Build history of the part. All positions in model axes, mm. A direction names the side the tool comes from. Round coordinates to 2 decimals unless told otherwise and drop trailing zeros. Order: outer loops, then holes, each group sorted by start corner. A loop starts at its lowest first (then second) coordinate and runs counter-clockwise, first axis right, second up. Notation, with made-up numbers: (17.25, -20.75) -> (22.25, -20.75) arc R19 ccw to (22.25, -2.75) -> close; hole circle Ø7 at (18, -37). An arc over 180 degrees is marked (long way). Use a Markdown table: item, result. Add a question column.
Item 1: Slice it at D-D, the plane z = 0. State how many separate pieces and enclosed holes the cut face has, plus the area to 3 significant figures.
Item 2: Probe L1, parallel to Z at x = -31.5, y = 0; L2, parallel to Z at x = 34, y = -15; L3, parallel to Y at x = 30.5, z = 2. List the from-to ranges inside material, lowest first.
Item 3: Two-plate mould, pull along Z, no slides. Class faces 5 (the face through (0, -5, -21)), 6 (the face through (-41, 20, -6)), 7 (the face through (37, 3, -3)): released by +Z, released by -Z, zero draft, split by the parting line, or undercut.
Item 4: Slice it at B-B, the plane y = -15. Give the cut face in (x, z).
Item 5: Slice it at A-A, the plane x = 35. Give the cut face in (y, z).
Item 6: 3-axis set-ups, long thin cutter, end or side, ignore diameter. For faces 1 (the face through (1.02, -4.59, -18.97)), 2 (the face through (31, -13, -4)), 3 (the face through (25, 0, 0)), 4 (the face through (-25, 0, 0)): which of +Z, -Z, +X, -X, +Y, -Y reach the whole face in a straight line?
Item 7: Pin check, flat tips, straight feed: pin 1 (4 mm diameter, centred on x = 35, z = 0, fed in from +Y); pin 2 (1.8 mm diameter, centred on x = 28.5, z = 1, fed in from -Y); pin 3 (7 mm diameter, centred on x = -37.5, z = 0.5, fed in from +Y). Stop position of each tip, or through.
Item 8: Slice it at C-C, the plane x = 0. Give the cut face in (y, z), plus the area to 3 significant figures.
from build123d import *

# Parameters (mm, degrees)
BODY_DEPTH             = 10
SKETCH14_R             = 7.5
BEARING_SUPPORT_DEPTH  = 7
SKETCH15_R             = 7.5
SKETCH15_R_2           = 4.7
BEARING_PLACE_DEPTH    = 4
SKETCH16_R             = 2
MOTOR_SHAFT_HOLE_DEPTH = 3
FILLET1_R              = 6
SKETCH17_R             = 7.25
SPRING_HOLE_DEPTH      = 10
SKETCH18_W             = 11
SKETCH18_H             = 6
NUT_HOLE_DEPTH         = 20
SKETCH19_R             = 3.25
SHAFT_HOLE_DEPTH       = 13
SKETCH20_R             = 4
BRAKE_SCREW_HOLE_DEPTH = 20
SKETCH21_W             = 6
SKETCH21_H             = 11
BRAKE_NUT_HOLE_DEPTH   = 20
CHAMFER1_SIZE          = 1


with BuildPart() as part:
    # Sketch1 → Body (new, symmetric)
    with BuildSketch(Plane.XY):
        Polygon((25, -25), (-25, -25), (-45, -25), (-45, 20), (-25, 20), (-25, 25), (25, 25), (25, 20), (45, 20), (45, -25), align=None)
    extrude(amount=BODY_DEPTH, both=True)

    # Sketch14 → Bearing_Support (add)
    with BuildSketch(Plane(origin=(0, 0, -10), x_dir=(-1, 0, 0), z_dir=(0, 0, -1))):
        Circle(SKETCH14_R)
    extrude(amount=BEARING_SUPPORT_DEPTH)

    # Sketch15 → Bearing_Place (add)
    with BuildSketch(Plane(origin=(0, 0, -17), x_dir=(-1, 0, 0), z_dir=(0, 0, -1))):
        Circle(SKETCH15_R)
        Circle(SKETCH15_R_2, mode=Mode.SUBTRACT)
    extrude(amount=BEARING_PLACE_DEPTH)

    # Sketch16 → Motor_Shaft_Hole (cut)
    with BuildSketch(Plane(origin=(0, 0, -17), x_dir=(-1, 0, 0), z_dir=(0, 0, -1))):
        Circle(SKETCH16_R)
    extrude(amount=-MOTOR_SHAFT_HOLE_DEPTH, mode=Mode.SUBTRACT)

    # Fillet1
    fillet1_edges = [part.edges().sort_by_distance(p)[0] for p in [
        (7.5, 0, -10),
    ]]
    fillet(fillet1_edges, radius=FILLET1_R)

    # Sketch17 → Spring_Hole (cut)
    with BuildSketch(Plane(origin=(0, 20, 0), x_dir=(1, 0, 0), z_dir=(0, 1, 0))):
        with Locations(Location((-35, 0, 0), (0, 0, 180))):
            Circle(SKETCH17_R)
    spring_hole = extrude(amount=-SPRING_HOLE_DEPTH, mode=Mode.SUBTRACT)

    # Sketch18 → Nut_Hole (cut)
    with BuildSketch(Plane.ZY.offset(45)):
        Rectangle(SKETCH18_W, SKETCH18_H)
    nut_hole = extrude(amount=-NUT_HOLE_DEPTH, mode=Mode.SUBTRACT)

    # Sketch19 → Shaft_Hole (cut)
    with BuildSketch(Plane(origin=(0, 10, 0), x_dir=(1, 0, 0), z_dir=(0, 1, 0))):
        with Locations(Location((-35, 0, 0), (0, 0, 180))):
            Circle(SKETCH19_R)
    shaft_hole = extrude(amount=-SHAFT_HOLE_DEPTH, mode=Mode.SUBTRACT)

    # Sketch20 → Brake_Screw_Hole (cut)
    with BuildSketch(Plane(origin=(45, 0, 0), x_dir=(0, 0, -1), z_dir=(1, 0, 0))):
        with Locations(Location((0, -15, 0), (0, 0, 90))):
            Circle(SKETCH20_R)
    brake_screw_hole = extrude(amount=-BRAKE_SCREW_HOLE_DEPTH, mode=Mode.SUBTRACT)

    # Sketch21 → Brake_Nut_Hole (cut)
    with BuildSketch(Plane.XZ.offset(25)):
        with Locations((28, 0)):
            Rectangle(SKETCH21_W, SKETCH21_H)
    brake_nut_hole = extrude(amount=-BRAKE_NUT_HOLE_DEPTH, mode=Mode.SUBTRACT)

    # Mirror1: Spring_Hole, Nut_Hole, Shaft_Hole, Brake_Screw_Hole, Brake_Nut_Hole across plane
    add(spring_hole.mirror(Plane(origin=(0, 0, 0), x_dir=(0, 0, 1), z_dir=(1, 0, 0))), mode=Mode.SUBTRACT)
    add(nut_hole.mirror(Plane(origin=(0, 0, 0), x_dir=(0, 0, 1), z_dir=(1, 0, 0))), mode=Mode.SUBTRACT)
    add(shaft_hole.mirror(Plane(origin=(0, 0, 0), x_dir=(0, 0, 1), z_dir=(1, 0, 0))), mode=Mode.SUBTRACT)
    add(brake_screw_hole.mirror(Plane(origin=(0, 0, 0), x_dir=(0, 0, 1), z_dir=(1, 0, 0))), mode=Mode.SUBTRACT)
    add(brake_nut_hole.mirror(Plane(origin=(0, 0, 0), x_dir=(0, 0, 1), z_dir=(1, 0, 0))), mode=Mode.SUBTRACT)

    # Chamfer1
    chamfer1_edges = [part.edges().sort_by_distance(p)[0] for p in [
        (25, 22.5, -10),
        (35, 20, -10),
        (-35, 20, 10),
        (-35, 20, -10),
        (-25, 22.5, -10),
        (0, 25, -10),
        (25, 25, 0),
        (25, 20, 0),
        (45, 20, 0),
        (-45, 20, 0),
        (-25, 20, 0),
        (-25, 25, 0),
        (35, 20, 10),
        (25, 22.5, 10),
        (0, 25, 10),
        (-27.75, 20, 0),
        (-25, 22.5, 10),
        (27.75, 20, 0),
    ]]
    chamfer(chamfer1_edges, length=CHAMFER1_SIZE)


solid = part.part
Check sheet entries:
| question | item | result |
|---|---|---|
| 1 | separate pieces | 5 |
| 1 | enclosed holes | 0 |
| 1 | area | 3,210 mm2 |
| 2 | L1 | -10 to -5.5, 5.5 to 10 |
| 2 | L2 | -10 to -4, 4 to 10 |
| 2 | L3 | -5 to -3, 3 to 10 |
| 3 | face 5 | released by -Z |
| 3 | face 6 | zero draft |
| 3 | face 7 | undercut |
| 4 | outline | (-45, -10) -> (45, -10) -> (45, -4) -> (31, -4) -> (31, -5.5) -> (25, -5.5) -> (25, 5.5) -> (31, 5.5) -> (31, 4) -> (45, 4) -> (45, 10) -> (-45, 10) -> (-45, 4) -> (-31, 4) -> (-31, 5.5) -> (-25, 5.5) -> (-25, -5.5) -> (-31, -5.5) -> (-31, -4) -> (-45, -4) -> close |
| 5 | outline | (-25, -10) -> (19, -10) -> (20, -9) -> (20, -8.25) -> (19, -7.25) -> (10, -7.25) -> (10, -3.25) -> (3, -3.25) -> (3, -5.5) -> (-3, -5.5) -> (-3, 5.5) -> (3, 5.5) -> (3, 3.25) -> (10, 3.25) -> (10, 7.25) -> (19, 7.25) -> (20, 8.25) -> (20, 9) -> (19, 10) -> (-25, 10) -> close; hole circle Ø8 at (-15, 0) |
| 6 | face 1 | -Z |
| 6 | face 2 | -Y |
| 6 | face 3 | +X |
| 6 | face 4 | -X |
| 7 | pin 1 | y = -3 |
| 7 | pin 2 | y = -5 |
| 7 | pin 3 | y = 10 |
| 8 | outline | (-25, -10) -> (-13.5, -10) arc R6 cw to (-7.5, -16) -> (-7.5, -21) -> (-4.7, -21) -> (-4.7, -17) -> (-2, -17) -> (-2, -14) -> (2, -14) -> (2, -17) -> (4.7, -17) -> (4.7, -21) -> (7.5, -21) -> (7.5, -16) arc R6 cw to (13.5, -10) -> (24, -10) -> (25, -9) -> (25, 9) -> (24, 10) -> (-25, 10) -> close |
| 8 | area | 1,130 mm2 |
